Autodesk Inventor part; units mm, degrees
ref_plane "YZ Plane" through (0, 0, 0) normal (1, 0, 0) x (0, 1, 0)
ref_plane "XZ Plane" through (0, 0, 0) normal (0, 1, 0) x (-1, 0, 0)
ref_plane "XY Plane" through (0, 0, 0) normal (0, 0, 1) x (1, 0, 0)
sketch "Skizze2" plane through (0, 0, 0) normal (0, 0, 1) x (1, 0, 0)
  line L0 (91, -66) -> (91, 215.3)
  line L1 (91, -66) -> (0, -66)
  line L2 (0, -66) -> (0, 0)
  line L3 (91, 215.3) -> (51, 215.3)
  line L4 (51, 215.3) -> (51, 174)
  line L5 (51, 174) -> (-39, 174)
  line L6 (-39, 174) -> (-39, 0)
  line L7 (-39, 0) -> (0, 0)
  line L8 (0, 0) -> (91, 0) construction
  dimension "d0" = 281.3
  dimension "d1" = 91
  dimension "d2" = 66
  dimension "d3" = 40
  dimension "d4" = 41.3
  dimension "d5" = 90
extrude "Extrusion1" add sketch "Skizze2" along normal blind 1
sketch "Skizze3" plane through (0, 0, 1) normal (0, 0, 1) x (1, 0, 0)
  circle A0 centre (4, -62) radius 1.5
  line L0 (0, -66) -> (91, -66)
  line L1 (0, 0) -> (0, -66)
  circle A1 centre (87.122, -62) radius 1.5
  line L2 (91, -66) -> (91, 215.3)
  circle A2 centre (-35, 4) radius 1.5
  line L3 (-39, 0) -> (0, 0)
  line L4 (-39, 174) -> (-39, 0)
  circle A3 centre (-35, 170) radius 1.5
  line L5 (51, 174) -> (-39, 174)
  dimension "d8" = 3
  dimension "d9" = 4
  dimension "d10" = 4
  dimension "d11" = 4
  dimension "d12" = 3
  dimension "d13" = 3.878
  dimension "d14" = 3
  dimension "d15" = 4
  dimension "d16" = 4
  dimension "d17" = 3
  dimension "d18" = 4
  dimension "d19" = 4
extrude "Extrusion2" cut sketch "Skizze3" against normal blind 1.5
sketch "Skizze5" plane through (0, 0, 0) normal (0, 0, -1) x (-1, 0, 0)
  line L0 (0, -66) -> (-91, -66)
  line L1 (-91, 215.3) -> (-51, 215.3)
  line L2 (-91, -66) -> (-89.5, -66)
  line L3 (-89.5, -66) -> (-89.5, 215.3)
  line L4 (-89.5, 215.3) -> (-91, 215.3)
  line L5 (-91, 215.3) -> (-91, -66)
  line L6 (-51, 215.3) -> (-51, 174)
  line L7 (-91, 215.3) -> (-51, 215.3)
  line L8 (-51, 215.3) -> (-51, 213.8)
  line L9 (-51, 213.8) -> (-91, 213.8)
  line L10 (-91, 213.8) -> (-91, 215.3)
  point P0 (0, 0)
  point P1 (-89.5, 213.8)
  dimension "d36" = 1.5
  dimension "d43" = 1.5
extrude "Extrusion4" add sketch "Skizze5" along normal blind 17.9
sketch "Skizze6" plane through (91, -66, 1) normal (1, 0, 0) x (0, 0, -1)
  line L0 (0, 0) -> (18.9, 0)
  line L1 (18.9, 0) -> (18.9, 279.8)
  line L2 (1, 0) -> (18.9, 0)
  line L3 (18.9, 0) -> (18.9, 6.5)
  line L4 (18.9, 6.5) -> (1, 6.5)
  line L5 (1, 6.5) -> (1, 0)
  line L6 (1, 279.8) -> (1, 0)
  line L7 (18.9, 0) -> (18.9, 279.8)
  line L8 (1, 0) -> (18.9, 0)
  line L9 (1, 279.8) -> (18.9, 279.8)
  point P0 (1, 66)
  point P1 (18.4, 281.3)
  dimension "d39" = 6.5
extrude "Extrusion5" cut sketch "Skizze6" against normal blind 1.5 contours L5 L4 L1 L0
fillet "Rundung1" radius 2 7 edges at (91, 74.65, 1) (91, 215.3, -8.45) (71, 215.3, 1) (51, 174, 0.5) (-39, 174, 0.5) (-39, 0, 0.5) (0, -66, 0.5)
sketch "Skizze7" plane through (0, 0, 1) normal (0, 0, 1) x (1, 0, 0)
  line L0 (89, 215.3) -> (51, 215.3)
  line L1 (91, -59.5) -> (91, 213.3)
  line L2 (49, 174) -> (-37, 174)
  line L3 (51, 213.3) -> (51, 176)
  point P0 (0, 0)
  point P1 (87, 211.3)
  point P2 (50, 170)
  dimension "d44" = 4
  dimension "d45" = 4
  dimension "d53" = 4
  dimension "d54" = 1
hole "Bohrung1" at (87, 211.3, 1) at (50, 170, 1) direction (0, 0, -1) diameter 3 depth 1
sketch "Skizze10" plane through (51, 215.3, -1) normal (0, 1, 0) x (1, 0, 0)
  line L0 (0, -1) -> (0, 16.9)
  line L1 (38.5, 16.9) -> (0, 16.9)
  line L2 (0, -1) -> (1.5, -1)
  line L3 (1.5, -1) -> (1.5, 16.9)
  line L4 (1.5, 16.9) -> (0, 16.9)
  line L5 (0, 16.9) -> (0, -1)
  point P0 (-51, -1)
  dimension "d58" = 1.5
extrude "Extrusion7" cut sketch "Skizze10" against normal up to surface (1.5 mm away)
properties part number "PCB_Qfab_Deckel"
The model under review builds one solid part; all positions refer to its coordinate system, in mm. A direction names the side the tool comes from. Coordinates: 2 decimals unless noted, no trailing zeros. Loops run counter-clockwise (first coordinate to the right, second up) from the corner with the lowest first, then second, coordinate; pieces in that order, holes last. Notation, with made-up numbers: (-38.5, 18.5) -> (-3.5, 18.5) arc R24 cw to (-3.5, 56.5) -> close; hole circle Ø11 at (19.25, 88.25). An arc over 180 degrees is marked (long way). Answer as CSV lines item,"result".
Item 1: Insertion check: pin 1 (3.5 mm diameter, centred on x = 87.122, y = -62, fed in from -Z); pin 2 (1.5 mm diameter, centred on y = 37, z = -9.5, fed in from -X); pin 3 (1.8 mm diameter, centred on x = 4, y = -62, fed in from +Z) (1 decimal); pin 4 (1.1 mm diameter, centred on y = 196.5, z = 0.5, fed in from -X). Each pin has a flat end and moves straight along its axis. Give the tip position at first contact, or say it passes through.
Results below:
pin 1,"stops at z = 0"
pin 2,"stops at x = 89.5"
pin 3,"passes through"
pin 4,"stops at x = 51"
Item 2: Take a section at A-A, the plane z = -8. State the section outline as (x, y) points, and give its area (3 significant figures).
Results below:
outline,"(52.5, 213.8) -> (89.5, 213.8) -> (89.5, -59.5) -> (91, -59.5) -> (91, 213.3) arc R2 ccw to (89, 215.3) -> (52.5, 215.3) -> close"
area,"467 mm2"
Item 3: Take a section at D-D, the plane x = 12. State the section outline as (y, z) points, and give its area (3 significant figures).
Results below:
outline,"(-66, 0) -> (174, 0) -> (174, 1) -> (-66, 1) -> close"
area,"240 mm2"
Item 4: For L1, parallel to Y at x = -35, z = 0.5; L2, parallel to X at y = 170, z = 0.8; L3, parallel to Y at x = 64, z = -10.75, list the stretches that pass through material, from the lowest coordinate up.
Results below:
L1,"y = 0 to 2.5, 5.5 to 168.5, 171.5 to 174"
L2,"x = -39 to -36.5, -33.5 to 48.5, 51.5 to 89.87"
L3,"y = 213.8 to 215.3"
Item 5: Take a section at C-C, the plane x = -12.5. State the section outline as (y, z) points.
Results below:
outline,"(0, 0) -> (174, 0) -> (174, 1) -> (0, 1) -> close"
Item 6: Take a section at B-B, the plane y = 67. State the section outline as (x, z) points, and give its area (3 significant figures).
Results below:
outline,"(-39, 0) -> (89.5, 0) -> (89.5, -17.9) -> (91, -17.9) -> (91, -1) arc R2 ccw to (89, 1) -> (-39, 1) -> close"
area,"156 mm2"
Item 7: Machinability: for faces 1 (the flat face through (71, 213.8, -9)), 2 (the flat face through (91, 75, -10)), which of the approach directions +Z, -Z, +X, -X, +Y, -Y give a long, thin tool a straight path to every point of the face, cutting with its end or side? Answer none if there is none.
Results below:
face 1,"-Z, -X, -Y"
face 2,"+Z, -Z, +X, +Y, -Y"
